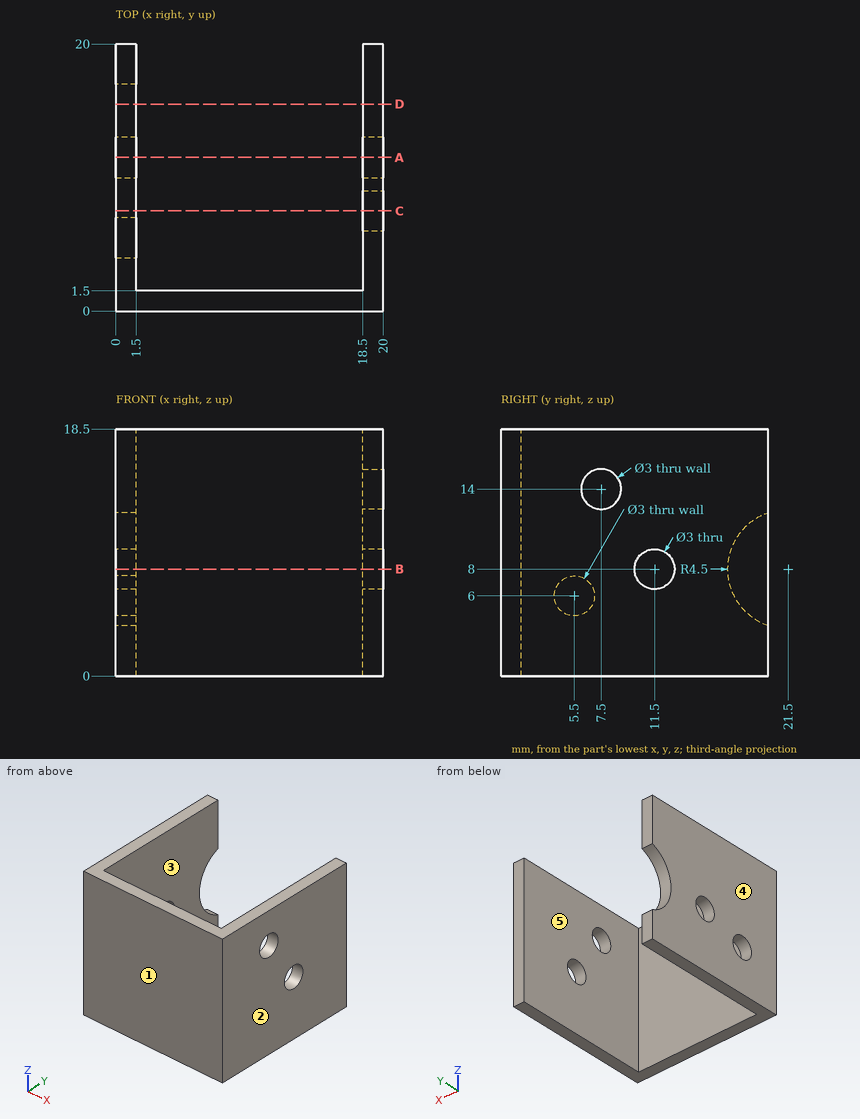
Drawing for the job (mm, zero at the part's lowest x, y, z). A direction names the side the tool comes from. Round coordinates to 2 decimals unless told otherwise and drop trailing zeros. Order: outer loops, then holes, each group sorted by start corner. A loop starts at its lowest first (then second) coordinate and runs counter-clockwise, first axis right, second up. Notation, with made-up numbers: M -6,-26 L 30,-26 A20 ccw 30,-14 Z; hole C 3,67.5 d11. An arc over 180 degrees is marked long. Use one line per item in the form item = value.
Q1. Probe L1, parallel to X at y = 9, z = 2.75; L2, parallel to Z at x = 0.5, y = 11.5; L3, parallel to Y at x = 19.3, z = 14. List the from-to ranges inside material, lowest first.
Recorded:
L1 = 0 to 1.5, 18.5 to 20
L2 = 0 to 6.5, 9.5 to 18.5
L3 = 0 to 6, 9 to 20
Q2. Which spindle directions (+Z, -Z, +X, -X, +Y, -Y) get a long thin tool onto all of the face, cutting with end or side? Do the marked faces 4 and 5. Say none if no direction does.
Recorded:
face_4 = +Z, -Z, -X, +Y, -Y
face_5 = +Z, -Z, +Y
Q3. Saw through at C-C on y = 7.5. Give the cut face in (x, z).
Recorded:
outline = M 0,0 L 1.5,0 L 1.5,18.5 L 0,18.5 Z; M 18.5,0 L 20,0 L 20,12.5 L 18.5,12.5 Z; M 18.5,15.5 L 20,15.5 L 20,18.5 L 18.5,18.5 Z
Q4. Saw through at D-D on y = 15.5. Give the cut face in (x, z).
Recorded:
outline = M 0,0 L 1.5,0 L 1.5,18.5 L 0,18.5 Z; M 18.5,0 L 20,0 L 20,18.5 L 18.5,18.5 Z
Q5. Saw through at B-B on z = 8. Give the cut face in (x, y).
Recorded:
outline = M 0,0 L 20,0 L 20,10 L 18.5,10 L 18.5,1.5 L 1.5,1.5 L 1.5,10 L 0,10 Z; M 0,13 L 1.5,13 L 1.5,17 L 0,17 Z; M 18.5,13 L 20,13 L 20,20 L 18.5,20 Z
Q6. Flat gauge pins, fed straight in: P1, Ø2, axis at x = 13.5, z = 11.5, coming from the +Y side; P2, Ø3.5, axis at y = 7.5, z = 14, coming from the +X side. Where does each tip first touch, or does it go through?
Recorded:
P1 = 1.5
P2 = 20
Q7. Saw through at A-A on y = 11.5. Give the cut face in (x, z).
Recorded:
outline = M 0,0 L 1.5,0 L 1.5,6.5 L 0,6.5 Z; M 0,9.5 L 1.5,9.5 L 1.5,18.5 L 0,18.5 Z; M 18.5,0 L 20,0 L 20,6.5 L 18.5,6.5 Z; M 18.5,9.5 L 20,9.5 L 20,18.5 L 18.5,18.5 Z
Q8. Two-plate mould, pull along X, no slides. Class the marked faces 1, 2 and 3: +X half, -X half, draft (parallel to the pull), parting line (faces both ways), or undercut.
Recorded:
face_1 = draft
face_2 = +X half
face_3 = undercut
